Work out the finished part from the listing and answer in its coordinate system (mm). Face numbers are marked on the shaded views. A direction names the side the tool comes from. Coordinates: 2 decimals unless noted, no trailing zeros. Order: outer loops, then holes, each group sorted by start corner. A loop starts at its lowest first (then second) coordinate and runs counter-clockwise, first axis right, second up.
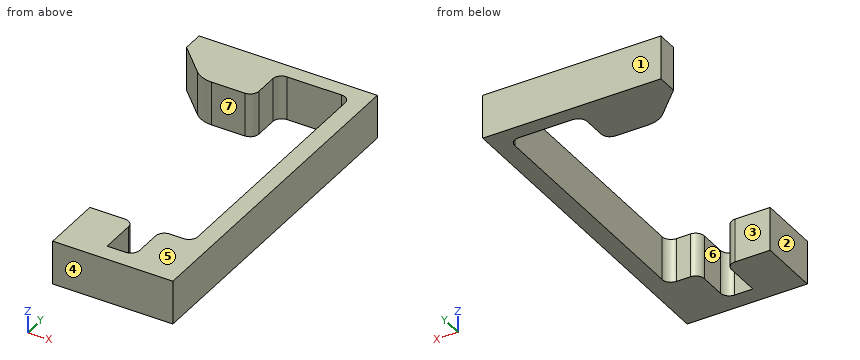
```python
from build123d import *

# Parameters (mm, degrees)
PAD_DEPTH    = 5
FILLET_R     = 1
FILLET001_R  = 1
CHAMFER_SIZE = 4
FILLET002_R  = 3
FILLET003_R  = 1


with BuildPart() as part:
    # Sketch (on CopyPart__Feature) → Pad (new body)
    with BuildSketch(Plane(origin=(211.803644, 488.825915, 357.796851), x_dir=(-1, 0, 0), z_dir=(0, 0, 1))):
        Polygon((3.2, 28.8), (-0.4, 28.8), (-0.4, -0.95), (7.85, -0.95), (7.85, 3.65), (17.92547, 3.65), (17.92547, -2.7), (7.85, -2.7), (-2.4, -2.7), (-2.4, 35.8), (11.3, 35.8), (11.3, 28.8), (6.3, 28.8), (6.3, 33.8), (3.2, 33.8), align=None)
    extrude(amount=PAD_DEPTH)

    # Fillet
    fillet_edges = [part.edges().sort_by_distance(p)[0] for p in [
        (203.953644, 489.775915, 360.296851),
        (212.203644, 489.775915, 360.296851),
        (212.203644, 460.025915, 360.296851),
        (205.503644, 460.025915, 360.296851),
    ]]
    fillet(fillet_edges, radius=FILLET_R)

    # Fillet001
    fillet001_edges = [part.edges().sort_by_distance(p)[0] for p in [
        (208.603644, 460.025915, 360.296851),
        (208.603644, 455.025915, 360.296851),
    ]]
    fillet(fillet001_edges, radius=FILLET001_R)

    # Chamfer
    chamfer_edges = [part.edges().sort_by_distance(p)[0] for p in [
        (193.878174, 485.175915, 360.296851),
    ]]
    chamfer(chamfer_edges, length=CHAMFER_SIZE)

    # Fillet002
    fillet002_edges = [part.edges().sort_by_distance(p)[0] for p in [
        (197.878174, 485.175915, 360.296851),
    ]]
    fillet(fillet002_edges, radius=FILLET002_R)

    # Fillet003
    fillet003_edges = [part.edges().sort_by_distance(p)[0] for p in [
        (203.953644, 485.175915, 360.296851),
    ]]
    fillet(fillet003_edges, radius=FILLET003_R)


solid = part.part
```
1. The part is cut by section B-B (z = 359.9). Determine the outline of the cut face in (x, y), plus the area to 3 significant figures.
2. For the marked faces 5, 6 and 7, determine the directions among +Z, -Z, +X, -X, +Y, -Y from which every point of the face is accessible in a straight line to the end or side of a thin tool.
3. Consider probe 1 along Y at (x, z) = (209.5, 360.7); probe 2 along Y at (x, z) = (207, 361); probe 3 along X at (y, z) = (457.5, 362.05). Determine where each line is inside the solid, lowest interval first.
4. The mould has two halves that part along Y. Classify the marked faces 1, 2, 3 and 4: released by +Y, released by -Y, zero draft, split by the parting line, or undercut.
5. Flat-ended cylindrical pins translate along their axes: pin 1 (2.5 mm diameter, centred on y = 457, z = 361, fed in from -X); pin 2 (10 mm diameter, centred on x = 205, y = 480.5, fed in from -Z). Find the tip coordinate at first contact, or state that the pin passes through.
6. The part is cut by section C-C (y = 470). Determine the outline of the cut face in (x, z), plus the area to 3 significant figures.
7. The part is cut by section A-A (x = 201). Determine the outline of the cut face in (y, z).
8. The part is cut by section D-D (x = 203.5). Determine the outline of the cut face in (y, z).
Worked out:
1. outline: (193.88, 489.18) - (197, 486.05) arc R3 ccw to (199.12, 485.18) - (202.95, 485.18) arc R1 ccw to (203.95, 486.18) - (203.95, 488.78) arc R1 cw to (204.95, 489.78) - (211.2, 489.78) arc R1 cw to (212.2, 488.78) - (212.2, 461.03) arc R1 cw to (211.2, 460.03) - (209.6, 460.03) arc R1 ccw to (208.6, 459.03) - (208.6, 456.03) arc R1 cw to (207.6, 455.03) - (205.5, 455.03) - (205.5, 459.03) arc R1 ccw to (204.5, 460.03) - (200.5, 460.03) - (200.5, 453.03) - (214.2, 453.03) - (214.2, 491.53) - (193.88, 491.53) - close
1. area: 214 mm2
2. face 5: +Z, +X, -X, +Y, -Y
2. face 6: +Z, -Z
2. face 7: +Z, -Z, -X
3. probe 1: y = 453.03 to 460.02, 489.78 to 491.53
3. probe 2: y = 453.03 to 455.03, 489.78 to 491.53
3. probe 3: x = 200.5 to 205.5, 208.6 to 214.2
4. face 1: released by +Y
4. face 2: zero draft
4. face 3: undercut
4. face 4: released by -Y
5. pin 1: stops at x = 200.5
5. pin 2: passes through
6. outline: (212.2, 357.8) - (214.2, 357.8) - (214.2, 362.8) - (212.2, 362.8) - close
6. area: 10.0 mm2
7. outline: (453.03, 357.8) - (460.03, 357.8) - (460.03, 362.8) - (453.03, 362.8) - close; (485.18, 357.8) - (491.53, 357.8) - (491.53, 362.8) - (485.18, 362.8) - close
8. outline: (453.03, 357.8) - (460.03, 357.8) - (460.03, 362.8) - (453.03, 362.8) - close; (485.34, 357.8) - (491.53, 357.8) - (491.53, 362.8) - (485.34, 362.8) - close
